Work out the finished part from the listing and answer in its coordinate system (mm). Face numbers are marked on the shaded views. A direction names the side the tool comes from. Round coordinates to 2 decimals unless told otherwise and drop trailing zeros. Write each loop counter-clockwise with the first axis right and the second up, starting at its lowest first coordinate (ties: lowest second). Pieces come first, ordered by that corner, then holes. Notation, with made-up numbers: (28.25, 33) -> (59.25, 33) arc R18 ccw to (59.25, 65) -> close; hole circle Ø1 at (5, 2). An arc over 180 degrees is marked (long way). One line per item, written item: value.
```python
from build123d import *


with BuildPart() as f1:
    # F0 (on Front) → F1 (revolve)
    with BuildSketch(Plane.XZ):
        with BuildLine():
            Line((0, 17.5), (0, 0))
            Line((0, 0), (60, 0))
            Line((60, 0), (60, 10))
            Line((60, 10), (75, 10))
            Line((75, 10), (75, 15))
            Line((75, 15), (72, 15))
            Line((72, 15), (72, 17.5))
            Line((72, 17.5), (67, 17.5))
            Line((67, 17.5), (67, 15))
            Line((67, 15), (50, 15))
            ThreePointArc((50, 15), (27.465305, 15.625482), (5, 17.5))
            Line((5, 17.5), (0, 17.5))
        make_face()
    revolve(axis=Axis((30, 0, 0), (1, 0, 0)))


solid = f1.part
```
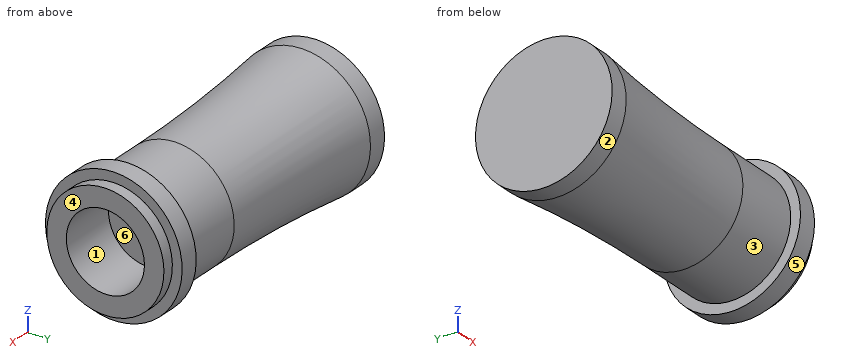
(1) For a pull along Z with two mould halves and no side action, classify the marked faces 4, 5 and 6 as pulls with the +Z half, pulls with the -Z half, needs draft (parallel to the pull), parting line crosses it, or undercut.
Reported:
face 4: needs draft
face 5: parting line crosses it
face 6: undercut
(2) Find section B-B on x = 63. Give the vertices of the cut face in (y, z), plus the area to 3 significant figures.
Reported:
outline: circle Ø30 at (0, 0); hole circle Ø20 at (0, 0)
area: 393 mm2
(3) A tool of negligible diameter and unlimited length cuts with its end or side. For the marked faces 1, 2 and 3, from which of +Z, -Z, +X, -X, +Y, -Y can it reach the whole face along a straight path? Write none if from no direction.
Reported:
face 1: +X
face 2: +X, -X
face 3: none
(4) Consider probe 1 along Y at (x, z) = (65, 0); probe 2 along Z at (x, y) = (69, 0). Determine where each line is inside the solid, lowest interval first.
Reported:
probe 1: y = -15 to -10, 10 to 15
probe 2: z = -17.5 to -10, 10 to 17.5
(5) Flat-ended cylindrical pins translate along their axes: pin 1 Ø6 at (x, z) = (44.5, 3.5) entering from +Y; pin 2 Ø8 at (x, y) = (42.5, -13.5) entering from +Z; pin 3 Ø10 at (x, y) = (32.5, -4.5) entering from -Z. Find the tip coordinate at first contact, or state that the pin passes through.
Reported:
pin 1: stops at y = 15.04
pin 2: stops at z = 11.7
pin 3: stops at z = -15.52
(6) Find section A-A on y = 0. Give the vertices of the cut face in (x, z), plus the area to 3 significant figures.
Reported:
outline: (0, -17.5) -> (5, -17.5) arc R406.25 cw to (50, -15) -> (67, -15) -> (67, -17.5) -> (72, -17.5) -> (72, -15) -> (75, -15) -> (75, -10) -> (60, -10) -> (60, 10) -> (75, 10) -> (75, 15) -> (72, 15) -> (72, 17.5) -> (67, 17.5) -> (67, 15) -> (50, 15) arc R406.25 cw to (5, 17.5) -> (0, 17.5) -> close
area: 2,070 mm2
(7) Find section D-D on x = 51. Give the vertices of the cut face in (y, z).
Reported:
outline: circle Ø30 at (0, 0)
